from build123d import *

# Parameters (mm, degrees)
BASE_FLANGE1_DEPTH      = 15.875
F_1_4_CLEARANCE_HOLE1_D = 6.7564
F_1_4_CLEARANCE_HOLE2_D = 6.7564
BOSS_EXTRUDE1_DEPTH     = 15.875
CUT_EXTRUDE1_DEPTH      = 49.098892269
BOSS_EXTRUDE2_DEPTH     = 1.5875
BOSS_EXTRUDE3_DEPTH     = 1.5875


# Read off the part's stored shape, not the designer's step: Base-Flange1
with BuildPart() as part:
    # Base-Flange1 outline → Base-Flange1 (new body)
    with BuildSketch(Plane(origin=(0, 0, 0), x_dir=(0, 0, -1), z_dir=(1, 0, 0))):
        with BuildLine():
            Line((1.5875, 0.79375), (1.5875, 26.9875))
            Line((1.5875, 26.9875), (0, 26.9875))
            Line((0, 26.9875), (0, 0.79375))
            ThreePointArc((0, 0.79375), (-0.232483992, 0.232483992), (-0.79375, 0))
            Line((-0.79375, 0), (-36.5125, 0))
            Line((-36.5125, 0), (-36.5125, -1.5875))
            Line((-36.5125, -1.5875), (-0.79375, -1.5875))
            ThreePointArc((-0.79375, -1.5875), (0.890048023, -0.890048023), (1.5875, 0.79375))
        make_face()
    extrude(amount=BASE_FLANGE1_DEPTH)

    # 1/4 Clearance Hole1 (through all)
    with Locations(Plane(origin=(0, 0, -1.5875), x_dir=(-1, 0, 0), z_dir=(0, 0, -1))):
        with Locations((-7.9375, 14.2875)):
            Hole(F_1_4_CLEARANCE_HOLE1_D / 2)

    # 1/4 Clearance Hole2 (through all)
    with Locations(Plane(origin=(0, 0, 0), x_dir=(1, 0, 0), z_dir=(0, 1, 0))):
        with Locations((7.9375, -23.8125)):
            Hole(F_1_4_CLEARANCE_HOLE2_D / 2)

    # Sketch11 → Boss-Extrude1 (add, through all)
    with BuildSketch(Plane(origin=(15.875, 0, 0), x_dir=(0, 0, -1), z_dir=(1, 0, 0))):
        with BuildLine():
            Line((1.5875, 0.79375), (1.5875, -1.5875))
            Line((1.5875, -1.5875), (-0.79375, -1.5875))
            ThreePointArc((-0.79375, -1.5875), (0.890048023, -0.890048023), (1.5875, 0.79375))
        make_face()
    extrude(amount=-BOSS_EXTRUDE1_DEPTH)

    # Sketch12 → Cut-Extrude1 (cut, through all)
    with BuildSketch(Plane(origin=(15.875, 0, 0), x_dir=(0, 0, -1), z_dir=(1, 0, 0))):
        with BuildLine():
            Line((-0.79375, 0), (0, 0))
            Line((0, 0), (0, 0.79375))
            ThreePointArc((0, 0.79375), (-0.232483992, 0.232483992), (-0.79375, 0))
        make_face()
    extrude(amount=-CUT_EXTRUDE1_DEPTH, mode=Mode.SUBTRACT)

    # Sketch13 → Boss-Extrude2 (add)
    with BuildSketch(Plane(origin=(15.875, 0, 0), x_dir=(0, 0, -1), z_dir=(1, 0, 0))):
        Polygon((0, 0), (0, 26.9875), (1.5875, 26.9875), (1.5875, -1.5875), (-36.5125, -1.5875), (-36.5125, 0), align=None)
    extrude(amount=-BOSS_EXTRUDE2_DEPTH)

    # Sketch14 → Boss-Extrude3 (add)
    with BuildSketch(Plane.ZY):
        Polygon((0, 0), (0, 26.9875), (-1.5875, 26.9875), (-1.5875, -1.5875), (36.5125, -1.5875), (36.5125, 0), align=None)
    extrude(amount=-BOSS_EXTRUDE3_DEPTH)


solid = part.part
Part model, mm, in its own coordinate system. A direction names the side the tool comes from. Coordinates: 2 decimals unless noted, no trailing zeros. Loops run counter-clockwise (first coordinate to the right, second up) from the corner with the lowest first, then second, coordinate; pieces in that order, holes last. Notation, with made-up numbers: (-15.5, 29.5) -> (17.5, 29.5) arc R20 ccw to (17.5, 34.5) -> close; hole circle Ø8 at (-14, 22). An arc over 180 degrees is marked (long way). Use a Markdown table: item, result. Add a question column.
Item 1: Band-saw the part on B-B on z = 25.5. Write the cut outline in (x, y) (1 decimal).
Item 2: Band-saw the part on D-D on y = 7.25. Write the cut outline in (x, z) (1 decimal), plus the area to 3 significant figures.
Item 3: Band-saw the part on A-A on y = 13.5. Write the cut outline in (x, z) (1 decimal), plus the area to 3 significant figures.
Item 4: Flat gauge pin, fed straight in: P1, Ø1, axis at x = 8.5, y = 23, coming from the +Z side. Where does the tip first touch, or does it go through?
Item 5: Pull direction Z, two halves, no side cores. Call faces 1 (the cylindrical face through (7.21, 10.99, -0.78)), 2 (the cylindrical face through (8.377, -0.805, 20.463)), 3 (the flat face through (8, -1, 36.512)): +Z half, -Z half, draft (parallel to the pull), parting line (faces both ways), or undercut.
Item 6: Band-saw the part on C-C on x = 8.75. Write the cut outline in (y, z), plus the area to 3 significant figures.
Item 7: Which spindle directions (+Z, -Z, +X, -X, +Y, -Y) get a long thin tool onto all of the face, cutting with end or side? Do faces 4 (the flat face through (8, 0, 19)), 5 (the flat face through (8, 10, -1.588)). Say none if no direction does.
Item 8: Probe probe 1 along Y at (x, z) = (1.25, 27.5). List the from-to ranges inside material, lowest first.
Geometry says:
| question | item | result |
|---|---|---|
| 1 | outline | (0, -1.6) -> (5, -1.6) -> (5, 0) -> (0, 0) -> close; (10.9, -1.6) -> (15.9, -1.6) -> (15.9, 0) -> (10.9, 0) -> close |
| 2 | outline | (0, -1.6) -> (15.9, -1.6) -> (15.9, 0) -> (0, 0) -> close |
| 2 | area | 25.2 mm² |
| 3 | outline | (0, -1.6) -> (4.7, -1.6) -> (4.7, 0) -> (0, 0) -> close; (11.2, -1.6) -> (15.9, -1.6) -> (15.9, 0) -> (11.2, 0) -> close |
| 3 | area | 14.8 mm² |
| 4 | P1 | z = 0 |
| 5 | face 1 | draft |
| 5 | face 2 | undercut |
| 5 | face 3 | +Z half |
| 6 | outline | (-1.59, -1.59) -> (11.01, -1.59) -> (11.01, 0) -> (0, 0) -> (0, 20.53) -> (-1.59, 20.53) -> close; (-1.59, 27.09) -> (0, 27.09) -> (0, 36.51) -> (-1.59, 36.51) -> close; (17.57, -1.59) -> (26.99, -1.59) -> (26.99, 0) -> (17.57, 0) -> close |
| 6 | area | 82.5 mm² |
| 7 | face 4 | +Z, +X, -X, +Y |
| 7 | face 5 | -Z, +X, -X, +Y, -Y |
| 8 | probe 1 | -1.59 to 0 |
